from build123d import *

# Parameters (mm, degrees)
SKETCH1_R           = 2.0319999999999987
SKETCH1_R_2         = 2.0320000000000005
BOSS_EXTRUDE1_DEPTH = 20.6375
FILLET1_R           = 6.35
BOSS_EXTRUDE2_START = 6.35
SKETCH3_R           = 2.159000000000005
BOSS_EXTRUDE2_DEPTH = 6.35
FILLET2_R           = 6.35
BOSS_EXTRUDE3_START = 20.6375
SKETCH4_R           = 2.032
BOSS_EXTRUDE3_DEPTH = 20.6375
FILLET3_R           = 3.175


with BuildPart() as part:
    # Sketch1 → Boss-Extrude1 (new body)
    with BuildSketch(Plane.XY):
        Polygon((0, 12.7), (0, 0), (11.112499999999999, -10.159999999999995), (38.1, -2.094157314500878), (38.1, 14.794157314500877), (11.112499999999999, 22.86), align=None)
        with Locations((11.112499999999999, 0)):
            Circle(SKETCH1_R, mode=Mode.SUBTRACT)
        with Locations((30.1625, 6.35)):
            Circle(SKETCH1_R_2, mode=Mode.SUBTRACT)
        with Locations((11.112499999999999, 12.7)):
            Circle(SKETCH1_R, mode=Mode.SUBTRACT)
    extrude(amount=BOSS_EXTRUDE1_DEPTH)

    # Fillet1
    fillet1_edges = [part.edges().sort_by_distance(p)[0] for p in [
        (0, 12.7, 10.31875),
        (11.112499999999999, 22.86, 10.31875),
        (38.1, 14.794157314500877, 10.31875),
        (38.1, -2.094157314500878, 10.31875),
        (11.112499999999999, -10.159999999999995, 10.31875),
        (0, 0, 10.31875),
    ]]
    fillet(fillet1_edges, radius=FILLET1_R)

    # Sketch3 → Boss-Extrude2 (add)
    with BuildSketch(Plane.XY.offset(20.6375).offset(BOSS_EXTRUDE2_START)):
        with BuildLine():
            Line((2.06521558288966, -1.888197104356259), (-32.77594211232474, 43.413196146372826))
            Line((-32.77594211232474, 43.413196146372826), (-32.77594211232474, 68.81319614637282))
            Line((-32.77594211232474, 68.81319614637282), (34.3497413303207, 17.639286263258136))
            ThreePointArc((34.3497413303207, 17.639286263258136), (37.1111008713377, 14.290641479729842), (38.1, 10.064460353186902))
            Line((38.1, 10.064460353186902), (38.1, 2.635539646813099))
            ThreePointArc((38.1, 2.635539646813099), (36.84259970760916, -1.157602614961311), (33.56836906517824, -3.448540722708889))
            Line((33.56836906517824, -3.448540722708889), (14.560051921917028, -9.129618843824993))
            ThreePointArc((14.560051921917028, -9.129618843824993), (11.324248271129079, -9.235318696210516), (8.456898439628453, -7.732021430517442))
            Line((8.456898439628453, -7.732021430517442), (2.06521558288966, -1.888197104356259))
        make_face()
        with Locations((1.57895919e-09, 31.151886065390322)):
            Circle(SKETCH3_R, mode=Mode.SUBTRACT)
    extrude(amount=-BOSS_EXTRUDE2_DEPTH)

    # Fillet2
    fillet2_edges = [part.edges().sort_by_distance(p)[0] for p in [
        (-32.77594211232474, 68.81319614637282, 23.812499999999996),
        (-32.77594211232474, 43.413196146372826, 23.812499999999996),
    ]]
    fillet(fillet2_edges, radius=FILLET2_R)

    # Sketch4 → Boss-Extrude3 (add)
    with BuildSketch(Plane(origin=(0, 0, 20.6375), x_dir=(-1, 0, 0), z_dir=(0, 0, -1)).offset(BOSS_EXTRUDE3_START)):
        with BuildLine():
            Line((32.77594211232474, 55.98737564555251), (32.77594211232474, 45.5726724047695))
            ThreePointArc((32.77594211232474, 45.5726724047695), (32.437811608681876, 43.52818587784627), (31.459430251294627, 41.701432660856774))
            Line((31.459430251294627, 41.701432660856774), (20.075942112324743, 26.900320790245356))
            Line((20.075942112324743, 26.900320790245356), (20.075942112324743, 59.13122909316789))
            Line((20.075942112324743, 59.13122909316789), (22.576114558777622, 61.03725958559999))
            ThreePointArc((22.576114558777622, 61.03725958559999), (29.243396196686703, 61.678109559777646), (32.77594211232474, 55.98737564555251))
        make_face()
        with Locations(Location((26.42594211232474, 55.98737564555251, 0), (0, 0, 180))):
            Circle(SKETCH4_R, mode=Mode.SUBTRACT)
        with Locations(Location((26.42594211232474, 45.5726724047695, 0), (0, 0, 180))):
            Circle(SKETCH4_R, mode=Mode.SUBTRACT)
    extrude(amount=-BOSS_EXTRUDE3_DEPTH)

    # Fillet3
    fillet3_edges = [part.edges().sort_by_distance(p)[0] for p in [
        (-20.075942112324743, 26.900320790245356, 10.31875),
    ]]
    fillet(fillet3_edges, radius=FILLET3_R)


solid = part.part
Input: part model. Units: mm. Frame: model coordinates. A direction names the side the tool comes from. Coordinates: 2 decimals unless noted, no trailing zeros. Order: outer loops, then holes, each group sorted by start corner. A loop starts at its lowest first (then second) coordinate and runs counter-clockwise, first axis right, second up.
1. Ray query, line 1 along Z through (x, y) = (8, 26); line 2 along Y through (x, z) = (33.5, 3.5); line 3 along X through (y, z) = (49.5, 12.5). Return the intervals inside material, ascending.
Checked values:
line 1: z = 20.64 to 26.99
line 2: y = -3.47 to 16.17
line 3: x = -32.78 to -20.08
2. Cut plane B-B, the plane y = 12.7. Return loops of the section in (x, z).
Checked values:
outline: (-9.15, 20.64) - (0.65, 20.64) - (0.65, 0) - (9.08, 0) - (9.08, 20.64) - (13.14, 20.64) - (13.14, 0) - (37.53, 0) - (37.53, 20.64) - (37.73, 20.64) - (37.73, 26.99) - (-9.15, 26.99) - close
3. Contact query for flat-ended pins moving along their axis: P1, Ø3, axis at x = -21, z = 19.5, coming from the +Y side; P2, Ø18, axis at x = 3.5, y = 32.5, coming from the -Z side; P3, Ø1, axis at y = 43, z = 8, coming from the +X side. Output: stop coordinate, or through.
Checked values:
P1: stops at y = 60.98
P2: stops at z = 20.64
P3: stops at x = -20.08
4. Cut plane C-C, the plane x = 30. Return loops of the section in (y, z).
Checked values:
outline: (-4.52, 0) - (4.32, 0) - (4.32, 20.64) - (8.38, 20.64) - (8.38, 0) - (17.22, 0) - (17.22, 20.64) - (20.96, 20.64) - (20.96, 26.99) - (-4.52, 26.99) - close
5. Cut plane A-A, the plane z = 12.25. Count the separate pieces of the cut face and the enclosed holes in it, plus the area to 3 significant figures.
Checked values:
separate pieces: 2
enclosed holes: 5
area: 1,160 mm2
6. Cut plane D-D, the plane x = -10. Return loops of the section in (y, z), plus the area to 3 significant figures.
Checked values:
outline: (13.8, 20.64) - (51.45, 20.64) - (51.45, 26.99) - (13.8, 26.99) - close
area: 239 mm2
7. Draft query along X for faces 5 (the cylindrical face through (-32.45, 43.56, 13.3)), 6 (the flat face through (24.2, -6.25, 13.68)), 7 (the flat face through (11, 0, 20.637)). Return one class per face: +X half, -X half, draft (parallel to the pull), parting line (faces both ways), or undercut.
Checked values:
face 5: -X half
face 6: +X half
face 7: undercut
8. Access query for faces 1 (the flat face through (-26, 56, 20.637)), 2 (the cylindrical face through (0.524, 12.429, 10.463)), 3 (the cylindrical face through (0.524, 0.271, 10.463)), 4 (the flat face through (24.2, 18.95, 10.17)). Directions: +Z, -Z, +X, -X, +Y, -Y. A direction counts if a zero-diameter tool reaches every point of the face in a straight line with its end or side. Return the directions, or none.
Checked values:
face 1: -Z
face 2: -Z, -X, +Y
face 3: -Z, -X, -Y
face 4: -Z, +X, +Y
